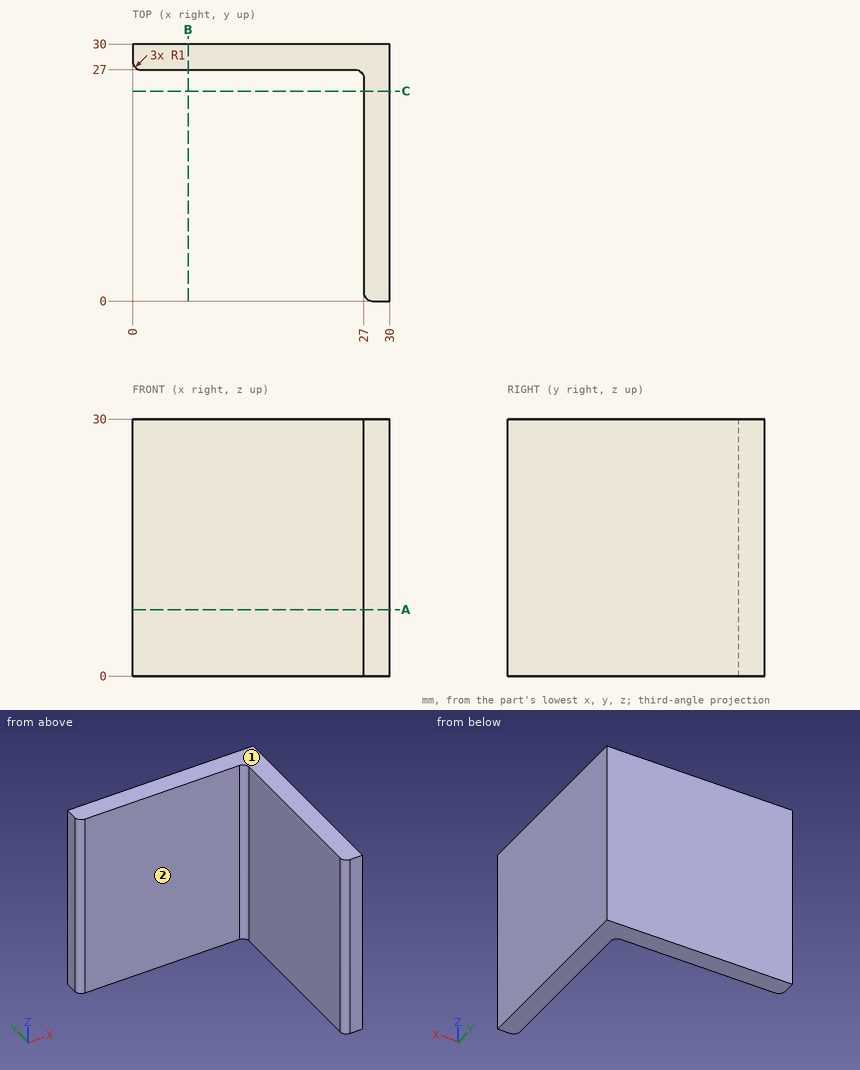
Job drawing, mm, ordinate dimensions from the low corner. One solid piece. A direction names the side the tool comes from. Give positions to 0.01 mm unless a question says otherwise; leave off trailing zeros. Loops run counter-clockwise (first coordinate to the right, second up) from the corner with the lowest first, then second, coordinate; pieces in that order, holes last. Notation, with made-up numbers: (34, -33) -> (45, -33) arc R17 ccw to (45, -2) -> close; hole circle Ø11 at (51.25, 86.5). An arc over 180 degrees is marked (long way). Use a Markdown table: item, result. Add a question column.
(1) Slice it at A-A on z = 7.75. List the corners of the cut face in (x, y).
(2) Slice it at B-B on x = 6.5. List the corners of the cut face in (y, z), and give its area (3 significant figures).
(3) Wall check: line 1 along Y through (x, z) = (20.75, 24.75); line 2 along Y through (x, z) = (27.25, 25.75). Give the ranges that are in metal, low to high.
(4) Drop flat-ended pins along their axis: pin 1 Ø12.5 at (x, z) = (9, 8) entering from -Y; pin 2 Ø12.5 at (y, z) = (17, 11.5) entering from -X. Give the stop position or say it passes through.
(5) Tool access for the marked faces 1 and 2: list every direction of +Z, -Z, +X, -X, +Y, -Y with a clear straight run to the whole face (end or side of a thin tool).
Filled sheet:
| question | item | result |
|---|---|---|
| 1 | outline | (0, 28) arc R1 ccw to (1, 27) -> (26, 27) arc R1 cw to (27, 26) -> (27, 1) arc R1 ccw to (28, 0) -> (30, 0) -> (30, 30) -> (0, 30) -> close |
| 2 | outline | (27, 0) -> (30, 0) -> (30, 30) -> (27, 30) -> close |
| 2 | area | 90.0 mm2 |
| 3 | line 1 | 27 to 30 |
| 3 | line 2 | 0.34 to 30 |
| 4 | pin 1 | y = 27 |
| 4 | pin 2 | x = 27 |
| 5 | face 1 | +Z, +X, -X, +Y, -Y |
| 5 | face 2 | +Z, -Z, -X, -Y |
